Design review of the part built by this model. Coordinates are the model's own, in mm. A direction names the side the tool comes from. Give positions to 0.01 mm unless a question says otherwise; leave off trailing zeros. Order: outer loops, then holes, each group sorted by start corner. A loop starts at its lowest first (then second) coordinate and runs counter-clockwise, first axis right, second up. Notation, with made-up numbers: (31.25, 47) -> (44.25, 47) arc R16 ccw to (44.25, 53) -> close; hole circle Ø8 at (89, -8.75). An arc over 180 degrees is marked (long way). One line per item, written item: value.
from build123d import *

# Parameters (mm, degrees)
SKETCH_1_R          = 8.5
EXTRUDE_1_DEPTH     = 28
SKETCH_2_R          = 7
CUT_EXTRUDE_3_DEPTH = 23
HOLE_WIZARD_M4_1_D  = 3.3
SKETCH_10_R         = 10.5
SKETCH_10_R_2       = 8.5
SKETCH_10_R_3       = 7
EXTRUDE_4_DEPTH     = 1
CHAMFER_1_SIZE      = 0.5


with BuildPart() as part:
    # 草图1 → 凸台-拉伸1 (new body)
    with BuildSketch(Plane.XY):
        Circle(SKETCH_1_R)
    extrude(amount=EXTRUDE_1_DEPTH)

    # 草图2 → 切除-拉伸3 (cut)
    with BuildSketch(Plane.XY.offset(28)):
        Circle(SKETCH_2_R)
    extrude(amount=-CUT_EXTRUDE_3_DEPTH, mode=Mode.SUBTRACT)

    # M4 螺纹孔1 (through all)
    with Locations(Plane(origin=(0, 0, 0), x_dir=(-1, 0, 0), z_dir=(0, 0, -1))):
        with Locations((0, 5), (0, 0), (-4.330127019, -2.5), (4.330127019, -2.5)):
            Hole(HOLE_WIZARD_M4_1_D / 2)

    # 草图10 → 凸台-拉伸4 (add)
    with BuildSketch(Plane.XY.offset(28)):
        Circle(SKETCH_10_R)
        Circle(SKETCH_10_R_2, mode=Mode.SUBTRACT)
        Circle(SKETCH_10_R_2)
        Circle(SKETCH_10_R_3, mode=Mode.SUBTRACT)
    extrude(amount=EXTRUDE_4_DEPTH)

    # 倒角1
    chamfer_1_edges = [part.edges().sort_by_distance(p)[0] for p in [
        (-8.5, 0, 0),
    ]]
    chamfer(chamfer_1_edges, length=CHAMFER_1_SIZE)


solid = part.part
Item 1: Clearance check with flat-ended pins moving along their axes: P1, Ø2, axis at x = 0, y = 0, coming from the -Z side; P2, Ø10, axis at x = 7.5, z = 20, coming from the +Y side; P3, Ø2, axis at y = -6.5, z = 14.5, coming from the -X side; P4, Ø3, axis at x = -1, z = 25, coming from the +Y side. State where each tip first meets the part, or that it passes through.
Returned:
P1: through
P2: y = 8.12
P3: x = -6.48
P4: y = 8.5
Item 2: Draft analysis for pull direction X (two halves, no side actions). For faces 1 (the cylindrical face through (10, 3.2, 28.5)), 2 (the flat face through (2, 0, 0)), 3 (the cylindrical face through (6.466, -2.681, 16.832)), state which applies: pulls with the +X half, pulls with the -X half, needs draft (parallel to the pull), parting line crosses it, or undercut.
Returned:
face 1: parting line crosses it
face 2: needs draft
face 3: undercut
Item 3: Add section B-B on y = 0. Give the boundary of the cut face in (x, z), plus the area to 3 significant figures.
Returned:
outline: (-10.5, 28) -> (-8.5, 28) -> (-8.5, 0.5) -> (-8, 0) -> (-1.65, 0) -> (-1.65, 5) -> (-7, 5) -> (-7, 29) -> (-10.5, 29) -> close; (1.65, 0) -> (8, 0) -> (8.5, 0.5) -> (8.5, 28) -> (10.5, 28) -> (10.5, 29) -> (7, 29) -> (7, 5) -> (1.65, 5) -> close
area: 144 mm²
Item 4: Machinability: for faces 4 (the cylindrical face through (4.57, 7.167, 14.058)), 5 (the flat face through (2, -7, 29)), 6 (the flat face through (0, 2, 5)), which of the approach directions +Z, -Z, +X, -X, +Y, -Y give a long, thin tool a straight path to every point of the face, cutting with its end or side? Answer none if there is none.
Returned:
face 4: -Z
face 5: +Z, +X, -X, +Y, -Y
face 6: +Z
Item 5: Add section D-D on y = -3.75. Count the separate pieces of the cut face and the enclosed holes in it, plus the area to 3 significant figures.
Returned:
separate pieces: 3
enclosed holes: 0
area: 141 mm²
Item 6: Add section A-A on x = 0. Give the boundary of the cut face in (y, z), plus the area to 3 significant figures.
Returned:
outline: (-10.5, 28) -> (-8.5, 28) -> (-8.5, 0.5) -> (-8, 0) -> (-1.65, 0) -> (-1.65, 5) -> (-7, 5) -> (-7, 29) -> (-10.5, 29) -> close; (1.65, 0) -> (3.35, 0) -> (3.35, 5) -> (1.65, 5) -> close; (6.65, 0) -> (8, 0) -> (8.5, 0.5) -> (8.5, 28) -> (10.5, 28) -> (10.5, 29) -> (7, 29) -> (7, 5) -> (6.65, 5) -> close
area: 128 mm²
Item 7: To check wall thickness, follow line 1 along Y through (x, z) = (0, 10.5); line 2 along Z through (x, y) = (5.5, -7.25); line 3 along Z through (x, y) = (5, 4). State the ranges of each line that lie inside material, in increasing order. Write a range as from..to.
Returned:
line 1: -8.5..-7, 7..8.5
line 2: 28..29
line 3: 0..5
Item 8: Add section C-C on z = 4.25. Give the boundary of the cut face in (x, y).
Returned:
outline: circle Ø17 at (0, 0); hole circle Ø3.3 at (-4.33, -2.5); hole circle Ø3.3 at (0, 0); hole circle Ø3.3 at (0, 5); hole circle Ø3.3 at (4.33, -2.5)
